Geometry: see drawing. Coordinates: mm, zero at the bounding-box minimum. A direction names the side the tool comes from. Round coordinates to 2 decimals unless told otherwise and drop trailing zeros. Write each loop counter-clockwise with the first axis right and the second up, starting at its lowest first coordinate (ties: lowest second). Pieces come first, ordered by that corner, then holes. Notation, with made-up numbers: M 69,51 L 125,51 A25 ccw 125,87 Z; hole C -22.75,-33.75 d9. An arc over 180 degrees is marked long. Use one line per item in the form item = value. Start each with the question number.
Item 1: Pin query (flat end, axial travel): pin 1 Ø2 at (y, z) = (18, 14.5) entering from -X; pin 2 Ø3 at (x, y) = (12.5, 5) entering from -Z. Return the tip coordinate at first contact, or that it passes through.
Item 2: Ray query, probe 1 along X at (y, z) = (18, 18.25) (1 decimal). Return the intervals inside material, ascending.
Item 3: Section query C-C (z = 16.5). Return loops of the section in (x, y) (1 decimal).
Item 4: Reachability of the marked faces 4 and 5 from +Z, -Z, +X, -X, +Y, -Y: full face, straight path, thin tool, end or side. Return the list, or none.
Item 5: Pull-direction query (X, two-part tool) for the marked faces 1, 2 and 3; classes: pulls with the +X half, pulls with the -X half, needs draft (parallel to the pull), parting line crosses it, or undercut.
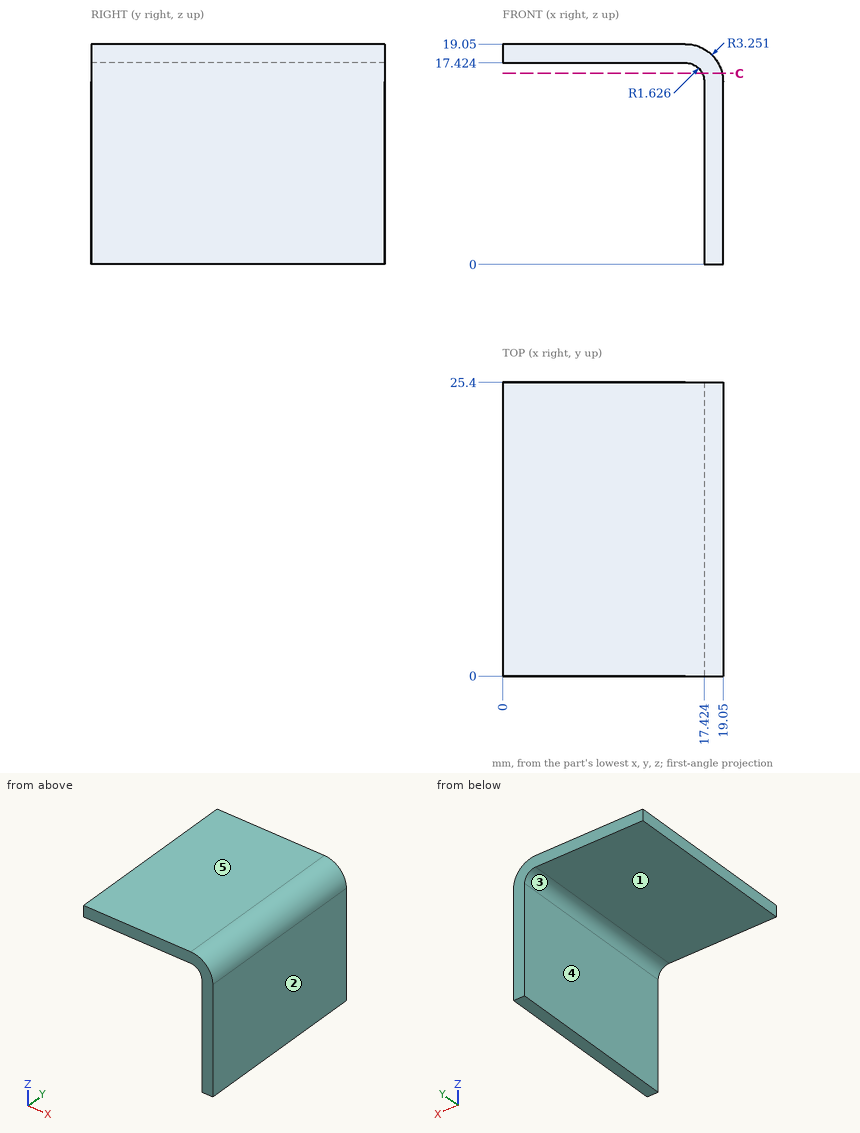
Working result:
q1.pin_1 = 17.42
q1.pin_2 = 17.42
q2.probe_1 = 0 to 17.9
q3.outline = M 17.3,0 L 19,0 L 19,25.4 L 17.3,25.4 Z
q4.face_4 = -Z, -X, +Y, -Y
q4.face_5 = +Z, +X, -X, +Y, -Y
q5.face_1 = needs draft
q5.face_2 = pulls with the +X half
q5.face_3 = pulls with the -X half
